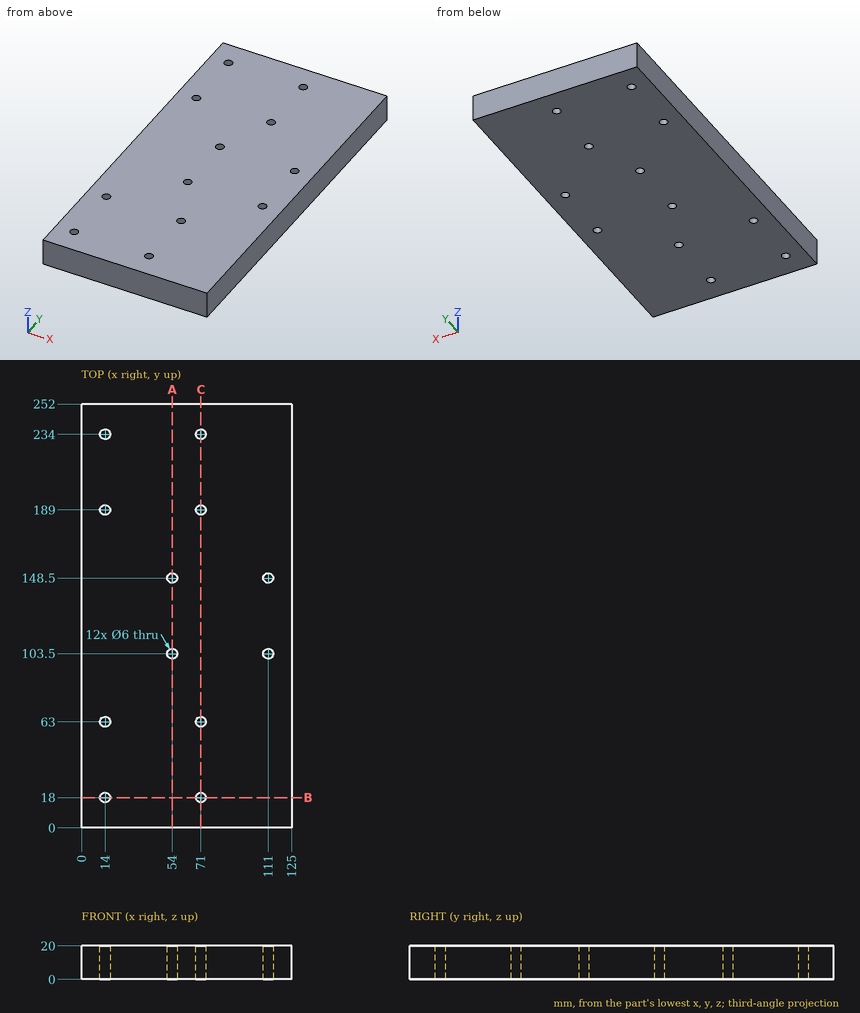
For this review, use the dimensioned drawing (mm, ordinates from the lowest corner) and the shaded views. Give positions to 0.01 mm unless a question says otherwise; leave off trailing zeros. Order: outer loops, then holes, each group sorted by start corner. A loop starts at its lowest first (then second) coordinate and runs counter-clockwise, first axis right, second up. Notation, with made-up numbers: M -7.5,55.5 L 4.5,55.5 A23 cw 4.5,75.5 Z; hole C 42.25,2 d5. An arc over 180 degrees is marked long. Use one line per item in the form item = value. Start each with the question number.
Item 1: We need section B-B on y = 18. Give the boundary of the cut face in (x, z).
Item 2: To check wall thickness, follow line 1 along X through (y, z) = (234, 10); line 2 along Y through (x, z) = (71, 13); line 3 along Y through (x, z) = (111, 5.5). State the ranges of each line that lie inside material, in increasing order. Write a range as from..to.
Item 3: We need section C-C on x = 71. Give the boundary of the cut face in (y, z).
Item 4: Insertion check: pin 1 Ø8 at (x, y) = (14, 189) entering from -Z; pin 2 Ø5 at (x, y) = (111, 148.5) entering from +Z. Each pin has a flat end and moves straight along its axis. Give the tip position at first contact, or say it passes through.
Item 5: We need section A-A on x = 54. Give the boundary of the cut face in (y, z).
Completed:
q1.outline = M 0,0 L 11,0 L 11,20 L 0,20 Z; M 17,0 L 68,0 L 68,20 L 17,20 Z; M 74,0 L 125,0 L 125,20 L 74,20 Z
q2.line_1 = 0..11, 17..68, 74..125
q2.line_2 = 0..15, 21..60, 66..186, 192..231, 237..252
q2.line_3 = 0..100.5, 106.5..145.5, 151.5..252
q3.outline = M 0,0 L 15,0 L 15,20 L 0,20 Z; M 21,0 L 60,0 L 60,20 L 21,20 Z; M 66,0 L 186,0 L 186,20 L 66,20 Z; M 192,0 L 231,0 L 231,20 L 192,20 Z; M 237,0 L 252,0 L 252,20 L 237,20 Z
q4.pin_1 = 0
q4.pin_2 = through
q5.outline = M 0,0 L 100.5,0 L 100.5,20 L 0,20 Z; M 106.5,0 L 145.5,0 L 145.5,20 L 106.5,20 Z; M 151.5,0 L 252,0 L 252,20 L 151.5,20 Z
